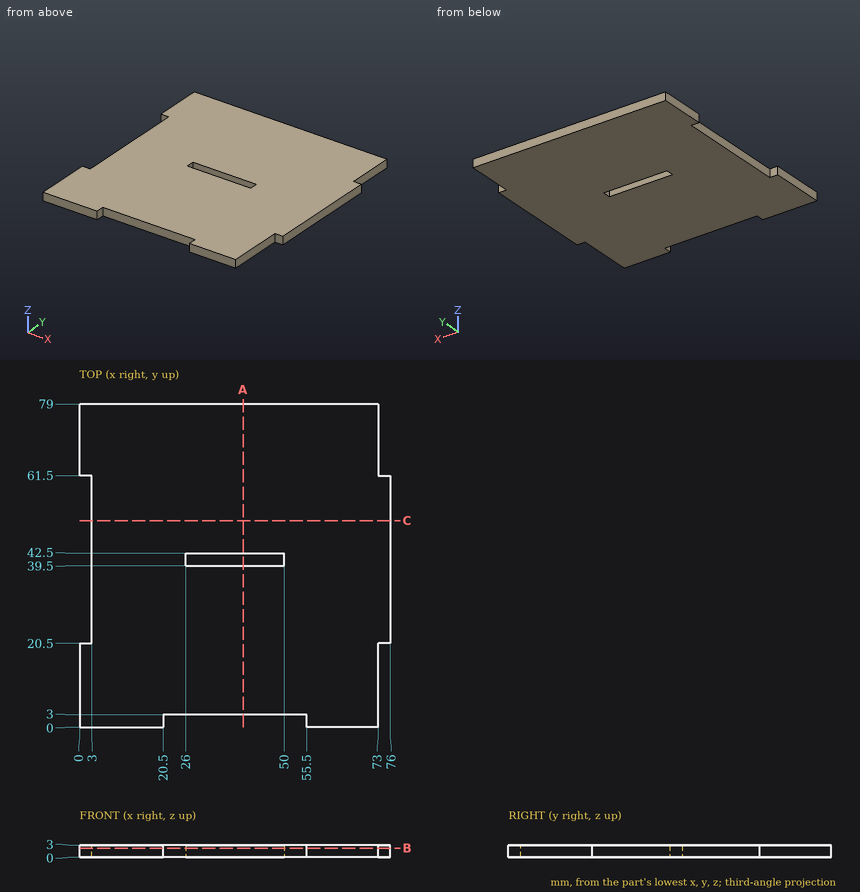
Geometry: see drawing. Coordinates: mm, zero at the bounding-box minimum. Coordinates: 2 decimals unless noted, no trailing zeros. Loops run counter-clockwise (first coordinate to the right, second up) from the corner with the lowest first, then second, coordinate; pieces in that order, holes last. Notation, with made-up numbers: (-1.75, 87) - (41.25, 87) arc R34 ccw to (41.25, 122) - close; hole circle Ø8 at (-37.5, -6). An arc over 180 degrees is marked (long way). Answer as CSV lines item,"result".
1. Section A-A (x = 40). Return loops of the section in (y, z), then the cut area to 3 significant figures.
Established:
outline,"(3, 0) - (39.5, 0) - (39.5, 3) - (3, 3) - close; (42.5, 0) - (79, 0) - (79, 3) - (42.5, 3) - close"
area,"219 mm2"
2. Ray query, line 1 (Y direction, x = 41.5, z = 0.75); line 2 (Y direction, x = 23.5, z = 2.8); line 3 (X direction, y = 6, z = 0.55). Return the intervals inside material, ascending.
Established:
line 1,"y = 3 to 39.5, 42.5 to 79"
line 2,"y = 3 to 79"
line 3,"x = 0 to 73"
3. Section C-C (y = 50.5). Return loops of the section in (x, z).
Established:
outline,"(3, 0) - (76, 0) - (76, 3) - (3, 3) - close"
4. Contact query for flat-ended pins moving along their axis: pin 1 (1 mm diameter, centred on x = 23.5, z = 0.5, fed in from -Y); pin 2 (1.5 mm diameter, centred on y = 1, z = 1, fed in from -X); pin 3 (0.9 mm diameter, centred on y = 12.5, z = 1.5, fed in from +X); pin 4 (0.9 mm diameter, centred on x = 75, z = 2, fed in from +Y). Output: stop coordinate, or through.
Established:
pin 1,"stops at y = 3"
pin 2,"stops at x = 0"
pin 3,"stops at x = 73"
pin 4,"stops at y = 61.5"
5. Section B-B (z = 2.25). Return loops of the section in (x, y).
Established:
outline,"(0, 0) - (20.5, 0) - (20.5, 3) - (55.5, 3) - (55.5, 0) - (73, 0) - (73, 20.5) - (76, 20.5) - (76, 61.5) - (73, 61.5) - (73, 79) - (0, 79) - (0, 61.5) - (3, 61.5) - (3, 20.5) - (0, 20.5) - close; hole (26, 39.5) - (50, 39.5) - (50, 42.5) - (26, 42.5) - close"
